from build123d import *

# Parameters (mm, degrees)
SKETCH1_R           = 25
BOSS_EXTRUDE1_DEPTH = 80
SKETCH2_R           = 10
BOSS_EXTRUDE2_DEPTH = 15
FILLET1_R           = 8
FILLET2_R           = 8
FILLET3_R           = 2
SKETCH3_R           = 5
CUT_EXTRUDE1_DEPTH  = 26


with BuildPart() as part:
    # Sketch1 → Boss-Extrude1 (new body)
    with BuildSketch(Plane.XY):
        Circle(SKETCH1_R)
    extrude(amount=BOSS_EXTRUDE1_DEPTH)

    # Sketch2 → Boss-Extrude2 (add)
    with BuildSketch(Plane.XY.offset(80)):
        Circle(SKETCH2_R)
    extrude(amount=BOSS_EXTRUDE2_DEPTH)

    # Fillet1
    fillet1_edges = [part.edges().sort_by_distance(p)[0] for p in [
        (-25, 0, 80),
    ]]
    fillet(fillet1_edges, radius=FILLET1_R)

    # Fillet2
    fillet2_edges = [part.edges().sort_by_distance(p)[0] for p in [
        (-25, 0, 0),
    ]]
    fillet(fillet2_edges, radius=FILLET2_R)

    # Fillet3
    fillet3_edges = [part.edges().sort_by_distance(p)[0] for p in [
        (-10, 0, 80),
        (-10, 0, 95),
    ]]
    fillet(fillet3_edges, radius=FILLET3_R)

    # Sketch3 → Cut-Extrude1 (cut)
    with BuildSketch(Plane.XY.offset(95)):
        Circle(SKETCH3_R)
    extrude(amount=-CUT_EXTRUDE1_DEPTH, mode=Mode.SUBTRACT)


solid = part.part
Source: CAD feature listing. Evaluate the final solid. Frame: model axes, mm. A direction names the side the tool comes from. Round coordinates to 2 decimals unless told otherwise and drop trailing zeros. Write each loop counter-clockwise with the first axis right and the second up, starting at its lowest first coordinate (ties: lowest second). Pieces come first, ordered by that corner, then holes. Notation, with made-up numbers: (24.25, -37.5) - (51.25, -37.5) arc R29 cw to (51.25, -0.5) - close; hole circle Ø6 at (-2.5, 2.5). An arc over 180 degrees is marked (long way). Use CSV: the item, a comma, the result in double quotes. Start each with the question number.
(1) Mould query, pull axis X, two halves, no side actions, for faces 1 (the face through (23.846, 7.509, 39.552)), 2 (the face through (0, 0, 0)), 3 (the face through (-1.08, -4.88, 82.18)). Classes: pulls with the +X half, pulls with the -X half, needs draft (parallel to the pull), parting line crosses it, or undercut.
(2) Cut plane A-A, the plane y = 0. Return loops of the section in (x, z).
(3) Material intervals for probe 1 along Z at (x, y) = (-2, 1); probe 2 along Z at (x, y) = (5.5, -12); probe 3 along Y at (x, z) = (0, 77) (3 decimals), sorted ascending. Write a range as [from, to].
(4) Set-up query: faces 4 (the face through (-2.17, -9.76, 87.42)), 5 (the face through (5.2, 0.1, 95)). Return all of +Z, -Z, +X, -X, +Y, -Y with unobstructed straight access to the full face (end or side cutting, diameter ignored); none if empty.
(5) Cut plane C-C, the plane z = 34. Return loops of the section in (x, y), and give its area (3 significant figures).
(6) First-contact query: pin 1 Ø2 at (x, y) = (-4.5, -13) entering from -Z; pin 2 Ø1.5 at (x, z) = (-10, 21) entering from +Y; pin 3 Ø1 at (x, z) = (-15, 76) entering from -Y; pin 4 Ø1.5 at (y, z) = (5, 14.5) entering from +X. Flat tips, straight axial feed; report the tip coordinate or a pass-through.
Geometry says:
1,face 1,"parting line crosses it"
1,face 2,"needs draft"
1,face 3,"undercut"
2,outline,"(-25, 8) arc R8 ccw to (-17, 0) - (17, 0) arc R8 ccw to (25, 8) - (25, 72) arc R8 ccw to (17, 80) - (12, 80) arc R2 cw to (10, 82) - (10, 93) arc R2 ccw to (8, 95) - (5, 95) - (5, 69) - (-5, 69) - (-5, 95) - (-8, 95) arc R2 ccw to (-10, 93) - (-10, 82) arc R2 cw to (-12, 80) - (-17, 80) arc R8 ccw to (-25, 72) - close"
3,probe 1,"[0, 69]"
3,probe 2,"[0, 80]"
3,probe 3,"[-23.245, -5], [5, 23.245]"
4,face 4,"+Z"
4,face 5,"+Z, +X, -X, +Y, -Y"
5,outline,"circle Ø50 at (0, 0)"
5,area,"1,960 mm²"
6,pin 1,"z = 0"
6,pin 2,"y = 23.23"
6,pin 3,"y = -19.17"
6,pin 4,"x = 24.64"
